```python
from build123d import *

# Parameters (mm, degrees)
BOSS_EXTRUDE1_DEPTH = 47.625
FILLET1_R           = 3.175
FILLET2_R           = 3.175
FILLET3_R           = 3.175


with BuildPart() as part:
    # Sketch2 → Boss-Extrude1 (new, symmetric)
    with BuildSketch(Plane.XY):
        Polygon((0, 0), (0, 76.2), (63.5, 76.2), (63.5, 57.15), (58.7375, 57.15), (58.7375, 71.4375), (4.7625, 71.4375), (4.7625, 4.7625), (31.75, 4.7625), (31.75, 0), align=None)
    extrude(amount=BOSS_EXTRUDE1_DEPTH, both=True)

    # Fillet1
    fillet1_edges = [part.edges().sort_by_distance(p)[0] for p in [
        (4.7625, 71.4375, 0),
    ]]
    fillet(fillet1_edges, radius=FILLET1_R)

    # Fillet2
    fillet2_edges = [part.edges().sort_by_distance(p)[0] for p in [
        (4.7625, 4.7625, 0),
    ]]
    fillet(fillet2_edges, radius=FILLET2_R)

    # Fillet3
    fillet3_edges = [part.edges().sort_by_distance(p)[0] for p in [
        (58.7375, 71.4375, 0),
    ]]
    fillet(fillet3_edges, radius=FILLET3_R)


solid = part.part
```
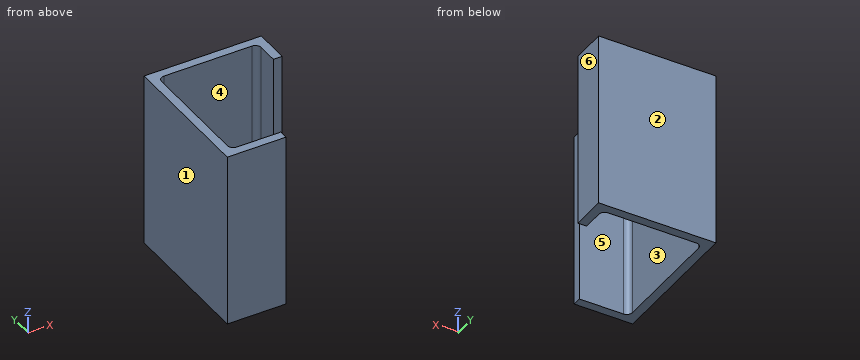
Check sheet for the modelled part. Datum: model origin and axes. Units: mm. Face numbers are marked on the shaded views. A direction names the side the tool comes from. Coordinates: 2 decimals unless noted, no trailing zeros. Order: outer loops, then holes, each group sorted by start corner. A loop starts at its lowest first (then second) coordinate and runs counter-clockwise, first axis right, second up. Notation, with made-up numbers: M 45,58.25 L 83,58.25 A30 cw 83,87.25 Z; hole C 34,57.25 d7. An arc over 180 degrees is marked long. One line per question, with ' | ' between items. Start each with the question number.
Item 1: Access from +Z, -Z, +X, -X, +Y, -Y to the whole of each face (thin tool, end or side, straight path). Record for the marked faces 4, 5 and 6.
Item 2: Sectioned sample at D-D on x = 38. Record the cut outline in (y, z) (1 decimal), and give its area (3 significant figures).
Item 3: Mould release check, pull along Y, two halves, no side actions. Record for the marked faces 1, 2 and 3: pulls with the +Y half, pulls with the -Y half, needs draft (parallel to the pull), parting line crosses it, or undercut.
Item 4: Sectioned sample at A-A on x = 14. Record the cut outline in (y, z) (1 decimal), and give its area (3 significant figures).
Item 5: Gauge pin test, flat ends, axial feed: P1, Ø8, axis at y = 13, z = 34.5, coming from the +X side; P2, Ø8, axis at x = 53, y = 65, coming from the -Z side; P3, Ø5, axis at y = 3, z = 20.5, coming from the +X side; P4, Ø1.4, axis at x = 62, z = 13, coming from the -Y side. Record the tip position at first contact, or that the pin passes through.
Item 6: Sectioned sample at C-C on y = 16.5. Record the cut outline in (x, z) (1 decimal).
Item 7: Material ranges on line 1 (Y direction, x = 8, z = -26.5); line 2 (X direction, y = 65, z = 12.5); line 3 (X direction, y = 19, z = 18), recorded low to high.
Answer below:
1) face 4: +Z, -Z | face 5: +Z, -Z, +X | face 6: +Z, -Z, +X, +Y, -Y
2) outline: M 71.4,-47.6 L 76.2,-47.6 L 76.2,47.6 L 71.4,47.6 Z | area: 454 mm^2
3) face 1: needs draft | face 2: pulls with the +Y half | face 3: undercut
4) outline: M 0,-47.6 L 4.8,-47.6 L 4.8,47.6 L 0,47.6 Z; M 71.4,-47.6 L 76.2,-47.6 L 76.2,47.6 L 71.4,47.6 Z | area: 907 mm^2
5) P1: stops at x = 4.76 | P2: passes through | P3: stops at x = 31.75 | P4: stops at y = 57.15
6) outline: M 0,-47.6 L 4.8,-47.6 L 4.8,47.6 L 0,47.6 Z
7) line 1: y = 0 to 4.76, 71.44 to 76.2 | line 2: x = 0 to 4.76, 58.74 to 63.5 | line 3: x = 0 to 4.76
